For this review, take the finished solid that the model builds, in its own axes (mm). A direction names the side the tool comes from. Coordinates: 2 decimals unless noted, no trailing zeros. Order: outer loops, then holes, each group sorted by start corner. A loop starts at its lowest first (then second) coordinate and runs counter-clockwise, first axis right, second up. Notation, with made-up numbers: (78.5, -34) -> (100.5, -34) arc R30 ccw to (100.5, 4) -> close; hole circle Ø9 at (27, -36.5). An arc over 180 degrees is marked (long way). Write item = value, one per line. Start each with the question number.
1) Wall thickness on probe 1 along Y at (x, z) = (15.25, 19); probe 2 along Y at (x, z) = (25.25, 17.5); probe 3 along Z at (x, y) = (26.25, -26.5): over which ranges is each line inside the solid? List them lowest first. Write a range as [from, to].
2) Draft analysis for pull direction Z (two halves, no side actions). For faces 1 (the face through (15.21, -29.828, 52.055)), 2 (the face through (15.21, -51.308, 26.834)), 3 (the face through (0, -39, 21)), state which applies: +Z half, -Z half, draft (parallel to the pull), parting line (faces both ways), or undercut.
3) Consider section D-D on y = -48. Give the boundary of the cut face in (x, z), and give its area (3 significant figures).
4) Consider section C-C on y = -31.5. Give the boundary of the cut face in (x, z), and give its area (3 significant figures).
5) Insertion check: pin 1 Ø1.5 at (x, z) = (4.5, 6.5) entering from +Y; pin 2 Ø4 at (x, z) = (8, 45) entering from -Y; pin 3 Ø6 at (x, z) = (10.5, 40.5) entering from -Y. Each pin has a flat end and moves straight along its axis. Give the tip position at first contact, or say it passes through.
6) Consider section B-B on z = 15. Give the boundary of the cut face in (x, y).
7) Machinability: for faces 4 (the face through (15.21, -68.96, 1.25)), 5 (the face through (15.21, -51.953, 18.715)), 6 (the face through (14.79, -38.183, 34.813)), which of the approach directions +Z, -Z, +X, -X, +Y, -Y give a long, thin tool a straight path to every point of the face, cutting with its end or side? Answer none if there is none.
from build123d import *

# Parameters (mm, degrees)
F4_DEPTH = 30
F5_R     = 3
F6_R     = 5
F7_DEPTH = 33.1
F8_R     = 4.37499


# Not quite as in the source:
# - a fillet or chamfer is up to 0.001 mm smaller than in the source, because OpenCascade refuses the exact size


with BuildPart() as f4:
    # F3 (on Right) → F4 (new body)
    with BuildSketch(Plane.YZ):
        Polygon((-70.8067866115, 0), (-5.9983764602, 0), (-30.002993414, 57.2861679354), (-45.3938998636, 15), (-53.6162102955, 17.9926762541), (-50.1960088622, 27.389602462), (-59.5929350701, 30.8098038952), align=None)
    extrude(amount=F4_DEPTH)

    # F5
    f5_edges = [f4.edges().sort_by_distance(p)[0] for p in [
        (15, -50.196009, 27.389602),
        (15, -30.002993, 57.286168),
        (15, -59.592935, 30.809804),
        (15, -70.806787, 0),
        (15, -5.998376, 0),
    ]]
    fillet(f5_edges, radius=F5_R)

    # F6 (on face) → F7 (cut)
    with BuildSketch(Plane.YZ.offset(30)):
        with Locations((-28.5474918187, 15)):
            Circle(F6_R)
    extrude(amount=-F7_DEPTH, mode=Mode.SUBTRACT)

    # F8 (radius 4.375 in the source; OpenCascade refuses exactly that, so slightly less here)
    f8_edges = [f4.edges().sort_by_distance(p)[0] for p in [
        (15, -53.61621, 17.992676),
        (15, -45.3939, 15),
    ]]
    fillet(f8_edges, radius=F8_R)


solid = f4.part
Answer sheet:
q1.probe_1 = [-63.89, -52.08], [-43.94, -31.55], [-25.55, -13.96]
q1.probe_2 = [-64.44, -51.09], [-44.93, -32.88], [-24.22, -13.33]
q1.probe_3 = [0, 10.44], [19.56, 48.93]
q2.face_1 = +Z half
q2.face_2 = undercut
q2.face_3 = draft
q3.outline = (0, 0) -> (30, 0) -> (30, 16.23) -> (0, 16.23) -> close
q3.area = 487 mm2
q4.outline = (0, 0) -> (30, 0) -> (30, 10.96) -> (0, 10.96) -> close; (0, 19.04) -> (30, 19.04) -> (30, 51.53) -> (0, 51.53) -> close
q4.area = 1,300 mm2
q5.pin_1 = -8.41
q5.pin_2 = -35.2
q5.pin_3 = -37.2
q6.outline = (0, -65.35) -> (30, -65.35) -> (30, -33.55) -> (0, -33.55) -> close; (0, -23.55) -> (30, -23.55) -> (30, -12.28) -> (0, -12.28) -> close
q7.face_4 = +X, -X, -Y
q7.face_5 = +X, -X
q7.face_6 = +Z, +X, -X
